Autodesk Fusion 360 part; units mm, degrees
sketch "Sketch1" plane through (0, 0, 0) normal (0, 0, 1) x (1, 0, 0)
  line L0 (0, 0) -> (55, 0)
  line L1 (67, 12) -> (67, 30)
  line L2 (55, 42) -> (0, 42)
  line L3 (0, 42) -> (0, 0)
  line L4 (67, 0) -> (55, 0) construction
  line L5 (55, 0) -> (55, 12) construction
  line L6 (55, 12) -> (67, 12) construction
  line L7 (67, 12) -> (67, 0) construction
  line L8 (67, 42) -> (55, 42) construction
  line L9 (55, 42) -> (55, 30) construction
  line L10 (55, 30) -> (67, 30) construction
  line L11 (67, 30) -> (67, 42) construction
  line L12 (55, 0) -> (67, 12)
  line L13 (55, 42) -> (67, 30)
  line L14 (0, 42) -> (13, 42)
  line L15 (13, 42) -> (13, 0)
  line L16 (13, 0) -> (0, 0)
  line L17 (0, 0) -> (0, 42)
  line L18 (13, 21) -> (67, 21)
  line L19 (67, 21) -> (13, 21)
  line L20 (13, 27) -> (67, 27)
  line L21 (67, 27) -> (67, 21)
  line L22 (13, 15) -> (67, 15)
extrude "Extrude1" add sketch "Sketch1" along normal blind 12
sketch "Sketch4" plane through (0, 0, 12) normal (0, 0, 1) x (-1, 0, 0)
  line L0 (-55, -42) -> (0, -42)
  line L1 (0, -42) -> (0, 0)
  line L2 (0, 0) -> (-55, 0)
  line L3 (-55, 0) -> (-67, -12)
  line L4 (-67, -12) -> (-67, -30)
  line L5 (-67, -30) -> (-55, -42)
  line L6 (0, -42) -> (-12, -42)
  line L7 (-12, -42) -> (-12, 0)
  line L8 (-12, 0) -> (0, 0)
  line L9 (0, 0) -> (0, -42)
extrude "Extrude2" add sketch "Sketch4" along normal blind 27 contours L0 L1 L2 L6 L7 L8 L9
sketch "Sketch5" plane through (0, 0, 39) normal (0, 0, 1) x (-1, 0, 0)
  line L0 (0, 0) -> (-12, 0)
  line L1 (-12, 0) -> (-12, -42)
  line L2 (-12, -42) -> (0, -42)
  line L3 (0, -42) -> (0, 0)
  line L4 (0, -42) -> (-12, -42)
  line L5 (-12, -42) -> (-12, 0)
  line L6 (-12, 0) -> (0, 0)
  line L7 (0, 0) -> (0, -42)
extrude "Extrude3" add sketch "Sketch5" along normal blind 21
fillet "Fillet1" radius 21 1 edges at (6, 0, 60)
sketch "Sketch6" plane through (0, 0, 0) normal (0, -1, 0) x (1, 0, 0)
  line L0 (12, 39) -> (0, 39)
  line L1 (0, 39) -> (0, 0)
  line L2 (0, 0) -> (55, 0)
  line L3 (55, 0) -> (55, 12)
  line L4 (55, 12) -> (12, 12)
  line L5 (12, 12) -> (12, 39)
  line L6 (0, 0) -> (0, 39)
  line L7 (0, 39) -> (12, 39)
fillet "Fillet2" radius 21 1 edges at (6, 42, 60)
sketch "Sketch7" plane through (0, 0, 12) normal (0, 0, 1) x (-1, 0, 0)
  line L0 (-12, -42) -> (-12, 0)
  line L1 (-12, 0) -> (-55, 0)
  line L2 (-55, 0) -> (-67, -12)
  line L3 (-67, -12) -> (-67, -30)
  line L4 (-67, -30) -> (-55, -42)
  line L5 (-55, -42) -> (-12, -42)
  line L6 (-25, -15) -> (-12, -15)
  line L7 (-25, -15) -> (-67, -15)
  line L8 (-67, -15) -> (-67, -27)
  line L9 (-67, -27) -> (-12, -27)
sketch "Sketch8" plane through (0, 0, 0) normal (0, -1, 0) x (1, 0, 0)
  line L0 (12, 12) -> (12, 54)
  line L1 (12, 54) -> (67, 12)
  line L2 (12, 12) -> (67, 12)
extrude "Extrude4" add sketch "Sketch8" against normal blind 27
sketch "Sketch9" plane through (0, 0, 0) normal (0, -1, 0) x (1, 0, 0)
  line L0 (12, 39) -> (0, 39)
  line L1 (0, 39) -> (0, 0)
  line L2 (0, 0) -> (55, 0)
  line L3 (55, 0) -> (55, 12)
  line L4 (55, 12) -> (67, 12)
  line L5 (67, 12) -> (12, 54)
  line L6 (12, 54) -> (12, 39)
  line L7 (12, 54) -> (12, 12)
  line L8 (12, 12) -> (67, 12)
  line L9 (12, 54) -> (67, 12)
extrude "Extrude5" cut sketch "Sketch9" against normal blind 15 contours L4 L5 L6 L7 L8 L9
CAD build for the part. Positions are in the model's coordinates, mm. A direction names the side the tool comes from. Coordinates: 2 decimals unless noted, no trailing zeros. Order: outer loops, then holes, each group sorted by start corner. A loop starts at its lowest first (then second) coordinate and runs counter-clockwise, first axis right, second up. Notation, with made-up numbers: (42.5, -18.5) - (61.5, -18.5) arc R22 cw to (61.5, 19.5) - close; hole circle Ø4 at (17, 10.25). An arc over 180 degrees is marked (long way). Answer in a Markdown table with one row per item.
1. Slice it at C-C, the plane y = 29. List the corners of the cut face in (x, z), then the cut area to 3 significant figures.
Answer:
| item | result |
|---|---|
| outline | (0, 0) - (67, 0) - (67, 12) - (12, 12) - (12, 58.42) - (0, 58.42) - close |
| area | 1,360 mm² |
2. Flat gauge pins, fed straight in: P1, Ø12.5, axis at x = 43.5, z = 24.5, coming from the +Y side; P2, Ø4, axis at y = 12, z = 53, coming from the +X side; P3, Ø8, axis at x = 50, y = 35, coming from the +Z side. Where does each tip first touch, or does it go through?
Answer:
| item | result |
|---|---|
| P1 | y = 27 |
| P2 | x = 12 |
| P3 | z = 12 |
3. Slice it at B-B, the plane z = 6. List the corners of the cut face in (x, y), then the cut area to 3 significant figures.
Answer:
| item | result |
|---|---|
| outline | (0, 0) - (55, 0) - (67, 12) - (67, 30) - (55, 42) - (0, 42) - close |
| area | 2,670 mm² |
4. Slice it at D-D, the plane z = 17. List the corners of the cut face in (x, y).
Answer:
| item | result |
|---|---|
| outline | (0, 0) - (12, 0) - (12, 15) - (60.45, 15) - (60.45, 27) - (12, 27) - (12, 42) - (0, 42) - close |
5. Drill centre lines: L1, parallel to X at y = 11, z = 35.5; L2, parallel to Y at x = 38, z = 16.5. Where is each one in solid material? Low to high. Write a range as from..to.
Answer:
| item | result |
|---|---|
| L1 | 0..12 |
| L2 | 15..27 |
6. Slice it at A-A, the plane x = 56. List the corners of the cut face in (y, z), then the cut area to 3 significant figures.
Answer:
| item | result |
|---|---|
| outline | (1, 0) - (41, 0) - (41, 12) - (27, 12) - (27, 20.4) - (15, 20.4) - (15, 12) - (1, 12) - close |
| area | 581 mm² |
7. 3-axis set-ups, long thin cutter, end or side, ignore diameter. For faces 1 (the face through (27, 15, 24)), 2 (the face through (39, 35, 12)), 3 (the face through (12, 30, 36)): which of +Z, -Z, +X, -X, +Y, -Y reach the whole face in a straight line?
Answer:
| item | result |
|---|---|
| face 1 | +Z, +X, -Y |
| face 2 | +Z, +X, +Y |
| face 3 | +Z, +X |
